```python
from build123d import *

# Parameters (mm, degrees)
CROQUIS1_W              = 34.35
CROQUIS1_H              = 29.5
CROQUIS1_R              = 2
SALIENTE_EXTRUIR1_DEPTH = 1.9
CROQUIS2_W              = 4
CROQUIS2_H              = 22
CORTAR_EXTRUIR2_DEPTH   = 1.6
REDONDEO1_R             = 1.5


with BuildPart() as part:
    # Croquis1 → Saliente-Extruir1 (new body)
    with BuildSketch(Plane(origin=(0, 0, 0), x_dir=(1, 0, 0), z_dir=(0, 1, 0))):
        with Locations((17.175, 14.75)):
            Rectangle(CROQUIS1_W, CROQUIS1_H)
        with Locations(Location((3.5, 3, 0), (0, 0, 90))):
            Circle(CROQUIS1_R, mode=Mode.SUBTRACT)
        with Locations(Location((30.85, 26.5, 0), (0, 0, 90))):
            Circle(CROQUIS1_R, mode=Mode.SUBTRACT)
    extrude(amount=SALIENTE_EXTRUIR1_DEPTH)

    # Croquis2 → Cortar-Extruir2 (cut)
    with BuildSketch(Plane(origin=(0, 1.9, 0), x_dir=(1, 0, 0), z_dir=(0, 1, 0))):
        with Locations((29.85, 11)):
            Rectangle(CROQUIS2_W, CROQUIS2_H)
        with Locations((4.5, 18.5)):
            Rectangle(CROQUIS2_W, CROQUIS2_H)
    extrude(amount=-CORTAR_EXTRUIR2_DEPTH, mode=Mode.SUBTRACT)

    # Redondeo1
    # the kernel refuses this fillet: 1.5 mm, written as the material it adds along each edge
    with BuildSketch(Plane(origin=(27.85, 1.9, -22), x_dir=(0, 0, 1), z_dir=(0, -1, 0))) as redondeo1_piece_1:
        with BuildLine():
            CenterArc((REDONDEO1_R, -REDONDEO1_R), REDONDEO1_R, 90, 90)
            Line((0, -REDONDEO1_R), (0, 0))
            Line((0, 0), (REDONDEO1_R, 0))
        make_face()
    extrude(amount=1.6)
    with BuildSketch(Plane(origin=(31.85, 1.9, -22), x_dir=(0, 0, 1), z_dir=(0, -1, 0)), Plane(origin=(2.5, 1.9, -7.5), x_dir=(0, 0, -1), z_dir=(0, -1, 0)), Plane(origin=(6.5, 1.9, -7.5), x_dir=(-1, 0, 0), z_dir=(0, -1, 0))) as redondeo1_piece_2:
        with BuildLine():
            CenterArc((REDONDEO1_R, REDONDEO1_R), REDONDEO1_R, 180, 90)
            Line((0, REDONDEO1_R), (0, 0))
            Line((0, 0), (REDONDEO1_R, 0))
        make_face()
    extrude(amount=1.6)
    # the kernel refuses this fillet: 1.5 mm, written as the material it takes off along each edge
    with BuildSketch(Plane(origin=(27.85, 5.65, 0), x_dir=(-1, 0, 0), z_dir=(0, -1, 0)), Plane(origin=(6.5, 5.65, -29.5), x_dir=(1, 0, 0), z_dir=(0, -1, 0))) as redondeo1_2_piece_1:
        with BuildLine():
            CenterArc((REDONDEO1_R, REDONDEO1_R), REDONDEO1_R, 180, 90)
            Line((0, REDONDEO1_R), (0, 0))
            Line((0, 0), (REDONDEO1_R, 0))
        make_face()
    extrude(amount=5.35, mode=Mode.SUBTRACT)
    with BuildSketch(Plane(origin=(31.85, 5.65, 0), x_dir=(1, 0, 0), z_dir=(0, -1, 0)), Plane(origin=(2.5, 5.65, -29.5), x_dir=(-1, 0, 0), z_dir=(0, -1, 0))) as redondeo1_2_piece_2:
        with BuildLine():
            CenterArc((REDONDEO1_R, -REDONDEO1_R), REDONDEO1_R, 90, 90)
            Line((0, -REDONDEO1_R), (0, 0))
            Line((0, 0), (REDONDEO1_R, 0))
        make_face()
    extrude(amount=5.35, mode=Mode.SUBTRACT)
    with BuildSketch(Plane(origin=(0, -3.75, -29.5), x_dir=(0, 0, 1), z_dir=(0, 1, 0)), Plane(origin=(0, -3.75, 0), x_dir=(1, 0, 0), z_dir=(0, 1, 0))) as redondeo1_2_piece_3:
        with BuildLine():
            CenterArc((REDONDEO1_R, REDONDEO1_R), REDONDEO1_R, 180, 90)
            Line((0, REDONDEO1_R), (0, 0))
            Line((0, 0), (REDONDEO1_R, 0))
        make_face()
    extrude(amount=9.4, mode=Mode.SUBTRACT)
    with BuildSketch(Plane(origin=(34.35, -3.75, -29.5), x_dir=(0, 0, 1), z_dir=(0, 1, 0)), Plane(origin=(34.35, -3.75, 0), x_dir=(-1, 0, 0), z_dir=(0, 1, 0))) as redondeo1_2_piece_4:
        with BuildLine():
            CenterArc((REDONDEO1_R, -REDONDEO1_R), REDONDEO1_R, 90, 90)
            Line((0, -REDONDEO1_R), (0, 0))
            Line((0, 0), (REDONDEO1_R, 0))
        make_face()
    extrude(amount=9.4, mode=Mode.SUBTRACT)


solid = part.part
```
Read the model definition and answer for the solid it produces. Units are mm, in the model's axes. A direction names the side the tool comes from. Round coordinates to 2 decimals unless told otherwise and drop trailing zeros. Loops run counter-clockwise (first coordinate to the right, second up) from the corner with the lowest first, then second, coordinate; pieces in that order, holes last. Notation, with made-up numbers: (11, -6) -> (23, -6) arc R34 cw to (23, 24) -> close; hole circle Ø4 at (62.25, 66). An arc over 180 degrees is marked (long way). One line per item, written item: value.
1) For faces 1 (the face through (32.624, 0.937, -27.423)), 2 (the face through (31.4, 1.11, -21.57)), 3 (the face through (5, 0.3, -18)), determine the directions among +Z, -Z, +X, -X, +Y, -Y from which every point of the face is accessible in a straight line to the end or side of a thin tool.
Answer list:
face 1: +Y, -Y
face 2: +Z, +Y
face 3: -Z, +Y
2) The mould has two halves that part along X. Classify faces 4 (the face through (0.43, 0.94, -0.45)), 5 (the face through (6.07, 1.11, -7.95)), 6 (the face through (17, 1.9, -15)): pulls with the +X half, pulls with the -X half, needs draft (parallel to the pull), parting line crosses it, or undercut.
Answer list:
face 4: pulls with the -X half
face 5: undercut
face 6: needs draft
3) Flat-ended cylindrical pins translate along their axes: P1, Ø2, axis at x = 4.5, z = -20.5, coming from the +Y side; P2, Ø0.5, axis at x = 29.5, y = 1, coming from the +Z side; P3, Ø0.8, axis at x = 4.5, y = 1, coming from the -Z side. Find the tip coordinate at first contact, or state that the pin passes through.
Answer list:
P1: stops at y = 0.3
P2: stops at z = -22
P3: stops at z = -7.5
4) Consider L1, parallel to X at y = 0.7, z = -26.5; L2, parallel to X at y = 1.85, z = -10.75; L3, parallel to X at y = 1.3, z = -22.5. Determine where each line is inside the solid, lowest interval first. Write a range as [from, to].
Answer list:
L1: x = [0, 2.5], [6.5, 28.85], [32.85, 34.35]
L2: x = [0, 2.5], [6.5, 27.85], [31.85, 34.35]
L3: x = [0, 2.5], [6.5, 34.35]
5) A cutting plane is placed at B-B (y = 1.5). Determine the outline of the cut face in (x, z), and give its area (3 significant figures).
Answer list:
outline: (0, -28) arc R1.5 ccw to (1.25, -29.48) arc R1.5 ccw to (2.5, -28) -> (2.5, -9) arc R1.5 cw to (4, -7.5) -> (5, -7.5) arc R1.5 cw to (6.5, -9) -> (6.5, -28) arc R1.5 ccw to (8, -29.5) -> (32.85, -29.5) arc R1.5 ccw to (34.35, -28) -> (34.35, -1.5) arc R1.5 ccw to (33.1, -0.02) arc R1.5 ccw to (31.85, -1.5) -> (31.85, -20.5) arc R1.5 cw to (30.35, -22) -> (29.35, -22) arc R1.5 cw to (27.85, -20.5) -> (27.85, -1.5) arc R1.5 ccw to (26.35, 0) -> (1.5, 0) arc R1.5 ccw to (0, -1.5) -> close; hole circle Ø4 at (3.5, -3); hole circle Ø4 at (30.85, -26.5)
area: 810 mm²
6) A cutting plane is placed at A-A (z = -26.5). Determine the outline of the cut face in (x, y).
Answer list:
outline: (0, 0) -> (28.85, 0) -> (28.85, 1.9) -> (6.5, 1.9) -> (6.5, 0.3) -> (2.5, 0.3) -> (2.5, 1.9) -> (0, 1.9) -> close; (32.85, 0) -> (34.35, 0) -> (34.35, 1.9) -> (32.85, 1.9) -> close
7) A cutting plane is placed at D-D (z = -18.5). Determine the outline of the cut face in (x, y), and give its area (3 significant figures).
Answer list:
outline: (0, 0) -> (34.35, 0) -> (34.35, 1.9) -> (31.85, 1.9) -> (31.85, 0.3) -> (27.85, 0.3) -> (27.85, 1.9) -> (6.5, 1.9) -> (6.5, 0.3) -> (2.5, 0.3) -> (2.5, 1.9) -> (0, 1.9) -> close
area: 52.5 mm²
8) A cutting plane is placed at C-C (x = 3.5). Determine the outline of the cut face in (y, z), and give its area (3 significant figures).
Answer list:
outline: (0, -29.5) -> (0.3, -29.5) -> (0.3, -7.59) -> (1.9, -7.59) -> (1.9, -5) -> (0, -5) -> close; (0, -1) -> (1.9, -1) -> (1.9, 0) -> (0, 0) -> close
area: 13.4 mm²
